The listing builds one solid part. Answer for the finished solid, in the listing's coordinates (mm). A direction names the side the tool comes from. Coordinates: 2 decimals unless noted, no trailing zeros. Write each loop counter-clockwise with the first axis right and the second up, starting at its lowest first coordinate (ties: lowest second). Pieces come first, ordered by that corner, then holes.
from build123d import *

# Parameters (mm, degrees)
SKETCH_1_W          = 80
SKETCH_1_H          = 24
EXTRUDE_1_DEPTH     = 6.5
SKETCH_2_W          = 6
SKETCH_2_H          = 3.5
EXTRUDE_2_DEPTH     = 1.5
SKETCH_3_W          = 3.260064366
SKETCH_3_H          = 1.448917496
EXTRUDE_3_DEPTH     = 1
SKETCH_4_R          = 2
CUT_EXTRUDE_1_DEPTH = 43.264050918
SKETCH_5_W          = 7
SKETCH_5_H          = 4.5
CUT_EXTRUDE_2_DEPTH = 6
SKETCH_6_W          = 28.5
SKETCH_6_H          = 13
CUT_EXTRUDE_3_DEPTH = 1.5
SKETCH_7_R          = 1.70863254
SKETCH_7_R_2        = 1.631149792
SKETCH_7_W          = 3.41726508
SKETCH_7_H          = 3.018578117
SKETCH_7_W_2        = 2.535605619
SKETCH_7_H_2        = 2.656348743
CUT_EXTRUDE_4_DEPTH = 1
FILLET_1_R          = 2


with BuildPart() as part:
    # 草图1 → 凸台-拉伸1 (new body)
    with BuildSketch(Plane(origin=(0, 0, 0), x_dir=(1, 0, 0), z_dir=(0, 1, 0))):
        Rectangle(SKETCH_1_W, SKETCH_1_H)
    extrude(amount=EXTRUDE_1_DEPTH)

    # 草图2 → 凸台-拉伸2 (add)
    with BuildSketch(Plane(origin=(0, 6.5, 0), x_dir=(1, 0, 0), z_dir=(0, 1, 0))):
        with Locations((0, 10.25)):
            Rectangle(SKETCH_2_W, SKETCH_2_H)
    extrude(amount=EXTRUDE_2_DEPTH)

    # 草图3 → 凸台-拉伸3 (add)
    with BuildSketch(Plane(origin=(0, 8, 0), x_dir=(1, 0, 0), z_dir=(0, 1, 0))):
        with Locations((0, 10.22231269)):
            Rectangle(SKETCH_3_W, SKETCH_3_H)
    extrude(amount=EXTRUDE_3_DEPTH)

    # 草图4 → 切除-拉伸1 (cut, through all)
    with BuildSketch(Plane(origin=(0, 6.5, 0), x_dir=(1, 0, 0), z_dir=(0, 1, 0))):
        with Locations(Location((-8, -8, 0), (0, 0, 270))):
            Circle(SKETCH_4_R)
        with Locations(Location((8, -8, 0), (0, 0, 270))):
            Circle(SKETCH_4_R)
        Polygon((-14.25, -12), (-14.25, 1), (-11.25, 1), (-11.25, -10.5), (11.25, -10.5), (11.25, 1), (14.25, 1), (14.25, -12), (11.25, -12), (-11.25, -12), align=None)
    extrude(amount=-CUT_EXTRUDE_1_DEPTH, mode=Mode.SUBTRACT)

    # 草图5 → 切除-拉伸2 (cut)
    with BuildSketch(Plane.XY.offset(12)):
        with Locations((-29.25, 2.75)):
            Rectangle(SKETCH_5_W, SKETCH_5_H)
        with Locations((29.25, 2.75)):
            Rectangle(SKETCH_5_W, SKETCH_5_H)
    extrude(amount=-CUT_EXTRUDE_2_DEPTH, mode=Mode.SUBTRACT)

    # 草图6 → 切除-拉伸3 (cut)
    with BuildSketch(Plane.XZ):
        with Locations((0, 5.5)):
            Rectangle(SKETCH_6_W, SKETCH_6_H)
    extrude(amount=-CUT_EXTRUDE_3_DEPTH, mode=Mode.SUBTRACT)

    # 草图7 → 切除-拉伸4 (cut)
    with BuildSketch(Plane.XZ):
        with Locations(Location((-32.962873036, -4.761215966, 0), (0, 0, 270))):
            Circle(SKETCH_7_R)
        with Locations(Location((-10.685766534, -4.761215966, 0), (0, 0, 270))):
            Circle(SKETCH_7_R_2)
        with Locations(Location((10.685766534, -4.761215966, 0), (0, 0, 90))):
            Circle(SKETCH_7_R_2)
        with Locations(Location((32.962873036, -4.761215966, 0), (0, 0, 90))):
            Circle(SKETCH_7_R)
        with Locations((-32.962873036, -9.409826265)):
            Rectangle(SKETCH_7_W, SKETCH_7_H)
        with Locations((-10.685766534, -8.98722533)):
            Rectangle(SKETCH_7_W_2, SKETCH_7_H_2)
        with Locations((10.685766534, -8.98722533)):
            Rectangle(SKETCH_7_W_2, SKETCH_7_H_2)
        with Locations((32.962873036, -9.409826265)):
            Rectangle(SKETCH_7_W, SKETCH_7_H)
    extrude(amount=-CUT_EXTRUDE_4_DEPTH, mode=Mode.SUBTRACT)

    # 圆角1
    fillet_1_edges = [part.edges().sort_by_distance(p)[0] for p in [
        (40, 3.25, 12),
        (-40, 3.25, 12),
        (-40, 3.25, -12),
        (40, 3.25, -12),
    ]]
    fillet(fillet_1_edges, radius=FILLET_1_R)


solid = part.part
Q1. The part is cut by section D-D, the plane z = 1.75. Write down the section's boundary in (x, y), then the cut area to 3 significant figures.
Answers below:
outline: (-40, 0) - (-14.25, 0) - (-14.25, 6.5) - (-40, 6.5) - close; (-11.25, 1.5) - (11.25, 1.5) - (11.25, 6.5) - (-11.25, 6.5) - close; (14.25, 0) - (40, 0) - (40, 6.5) - (14.25, 6.5) - close
area: 447 mm2
Q2. The part is cut by section B-B, the plane y = 3.75. Write down the section's boundary in (x, z), then the cut area to 3 significant figures.
Answers below:
outline: (-40, -10) arc R2 ccw to (-38, -12) - (38, -12) arc R2 ccw to (40, -10) - (40, 10) arc R2 ccw to (38, 12) - (32.75, 12) - (32.75, 6) - (25.75, 6) - (25.75, 12) - (14.25, 12) - (14.25, -1) - (11.25, -1) - (11.25, 10.5) - (-11.25, 10.5) - (-11.25, -1) - (-14.25, -1) - (-14.25, 12) - (-25.75, 12) - (-25.75, 6) - (-32.75, 6) - (-32.75, 12) - (-38, 12) arc R2 ccw to (-40, 10) - close; hole circle Ø4 at (-8, 8); hole circle Ø4 at (8, 8)
area: 1,700 mm2
Q3. Which of the six approach directions +Z, -Z, +X, -X, +Y, -Y give full straight-line access (tool end or side, diameter ignored) to faces 4 (the face through (0, 4, 10.5)), 5 (the face through (33, 1, -9)), 6 (the face through (32.75, 3, 9)), 7 (the face through (3, 7, -10)), 8 (the face through (-3, 7, -10))?
Answers below:
face 4: +Z, +Y, -Y
face 5: -Y
face 6: +Z
face 7: +Z, -Z, +X, +Y
face 8: +Z, -Z, -X, +Y
Q4. The part is cut by section A-A, the plane z = 8. Write down the section's boundary in (x, y).
Answers below:
outline: (-40, 0) - (-14.25, 0) - (-14.25, 6.5) - (-40, 6.5) - close; (-11.25, 1.5) - (-10, 1.5) - (-10, 6.5) - (-11.25, 6.5) - close; (-6, 1.5) - (6, 1.5) - (6, 6.5) - (-6, 6.5) - close; (10, 1.5) - (11.25, 1.5) - (11.25, 6.5) - (10, 6.5) - close; (14.25, 0) - (40, 0) - (40, 6.5) - (14.25, 6.5) - close; hole (-32.75, 0.5) - (-25.75, 0.5) - (-25.75, 5) - (-32.75, 5) - close; hole (25.75, 0.5) - (32.75, 0.5) - (32.75, 5) - (25.75, 5) - close
Q5. The part is cut by section C-C, the plane x = -8. Write down the section's boundary in (y, z), then the cut area to 3 significant figures.
Answers below:
outline: (0, -12) - (6.5, -12) - (6.5, 6) - (1.5, 6) - (1.5, -1) - (0, -1) - close; (1.5, 10) - (6.5, 10) - (6.5, 10.5) - (1.5, 10.5) - close
area: 109 mm2
Q6. Find the intervals of material crossed by probe 1 along X at (y, z) = (2.5, 1.5); probe 2 along Z at (x, y) = (11, 0.75); probe 3 along Y at (x, z) = (-26.5, 9), in increasing order.
Answers below:
probe 1: x = -40 to -14.25, -11.25 to 11.25, 14.25 to 40
probe 2: z = -12 to -10.32, -7.66 to -6.36, -3.16 to -1
probe 3: y = 0 to 0.5, 5 to 6.5
Q7. Given pin 1 (6 mm diameter, centred on x = 24, z = -9, fed in from +Y); pin 2 (4 mm diameter, centred on x = 13.5, y = 7.5, fed in from -Z); pin 3 (0.8 mm diameter, centred on x = 0, y = 8.5, fed in from +Z); pin 4 (2.5 mm diameter, centred on x = 10.69, z = -4.76, fed in from -Y), each flat-ended and moving along its own axis, determine where each tip first touches the part or whether it passes through.
Answers below:
pin 1: stops at y = 6.5
pin 2: stops at z = -12
pin 3: stops at z = -9.5
pin 4: stops at y = 1
Q8. Determine the mould class of faces 1 (the face through (-24, 3, 12)), 2 (the face through (0, 1.5, 5)), 3 (the face through (25.75, 3, 9)) for opening direction Y: released by +Y, released by -Y, zero draft, split by the parting line, or undercut.
Answers below:
face 1: zero draft
face 2: released by -Y
face 3: undercut
